```python
from build123d import *

# Parameters (mm, degrees)
CROQUIS1_R              = 2
CROQUIS1_R_2            = 3.5
CROQUIS1_R_3            = 4
CROQUIS1_W              = 30
CROQUIS1_H              = 3
CROQUIS1_R_4            = 1.5
CROQUIS1_W_2            = 15
CROQUIS1_H_2            = 55
SALIENTE_EXTRUIR4_DEPTH = 3


with BuildPart() as part:
    # Croquis1 → Saliente-Extruir4 (new body)
    with BuildSketch(Plane.XY):
        Polygon((-190, 67.5), (-190, -67.5), (-97.5, -67.5), (-97.5, -70.5), (-67.5, -70.5), (-67.5, -67.5), (-15, -67.5), (-15, -70.5), (15, -70.5), (15, -67.5), (67.5, -67.5), (67.5, -70.5), (97.5, -70.5), (97.5, -67.5), (190, -67.5), (190, 67.5), align=None)
        with Locations((-119.3, -56.25)):
            Circle(CROQUIS1_R, mode=Mode.SUBTRACT)
        with Locations((-170, -37.5)):
            Circle(CROQUIS1_R_2, mode=Mode.SUBTRACT)
        with Locations((-139.5, -47.5)):
            Circle(CROQUIS1_R_3, mode=Mode.SUBTRACT)
        with Locations((-119.3, -38.75)):
            Circle(CROQUIS1_R, mode=Mode.SUBTRACT)
        with Locations((-82.5, -29)):
            Rectangle(CROQUIS1_W, CROQUIS1_H, mode=Mode.SUBTRACT)
        with Locations((170, -37.5)):
            Circle(CROQUIS1_R_2, mode=Mode.SUBTRACT)
        with Locations((0, -29)):
            Rectangle(CROQUIS1_W, CROQUIS1_H, mode=Mode.SUBTRACT)
        with Locations((82.5, -29)):
            Rectangle(CROQUIS1_W, CROQUIS1_H, mode=Mode.SUBTRACT)
        with Locations((-22, 9.5)):
            Circle(CROQUIS1_R_4, mode=Mode.SUBTRACT)
        with Locations((0, 25)):
            Rectangle(CROQUIS1_W_2, CROQUIS1_H_2, mode=Mode.SUBTRACT)
        with Locations((-167.5, 39.5)):
            Circle(CROQUIS1_R_4, mode=Mode.SUBTRACT)
        Polygon((-180, 57.5), (-180, 64.5), (-155, 64.5), (-155, 57.5), (-163.4, 57.5), (-173.4, 57.5), align=None, mode=Mode.SUBTRACT)
        with Locations((-22, 45.5)):
            Circle(CROQUIS1_R_4, mode=Mode.SUBTRACT)
        Polygon((-19.6, 57.5), (-19.6, 64.5), (5.4, 64.5), (5.4, 57.5), (-3, 57.5), (-3, 54.5), (-13, 54.5), (-13, 57.5), align=None, mode=Mode.SUBTRACT)
        with Locations((167.5, 39.5)):
            Circle(CROQUIS1_R_4, mode=Mode.SUBTRACT)
        Polygon((155, 57.5), (155, 64.5), (180, 64.5), (180, 57.5), (171.6, 57.5), (161.6, 57.5), align=None, mode=Mode.SUBTRACT)
    extrude(amount=SALIENTE_EXTRUIR4_DEPTH)


solid = part.part
```
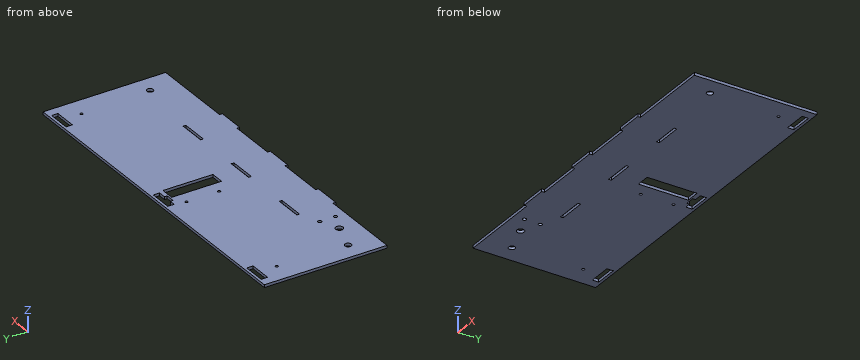
Could you check a few things on this model? Use its own coordinates, in mm. Coordinates: 2 decimals unless noted, no trailing zeros. Write each loop counter-clockwise with the first axis right and the second up, starting at its lowest first coordinate (ties: lowest second). Pieces come first, ordered by that corner, then holes. Notation, with made-up numbers: (6.5, 11.25) -> (49.5, 11.25) arc R13 cw to (49.5, 27.25) -> close; hole circle Ø2 at (-12.75, 3). An arc over 180 degrees is marked (long way). One line per question, with ' | ' between items. Start each with the question number.
1. If we section it at A-A (y = 24.5): Please give me the cut outline in (x, z).
2. If we section it at D-D (x = -106): Please give me the cut outline in (y, z).
3. Please list where these lines run through material, in increasing order: line 1 along Y through (x, z) = (-119.3, 0.75); line 2 along Y through (x, z) = (-170, 1.35); line 3 along Y through (x, z) = (-6, 1.2).
4. If we section it at C-C (y = -47.5): Please give me the cut outline in (x, z).
5. If we section it at B-B (z = 0.6): Count the separate pieces of the cut face and the enclosed holes in it, and give its area (3 significant figures).
6. Will these pins go through, and if not, where does the flat tip stop? P1, Ø1.5, axis at y = -68.5, z = 2, coming from the +X side; P2, Ø1, axis at x = -149.5, z = 1, coming from the -Y side.
Return value:
1) outline: (-190, 0) -> (-7.5, 0) -> (-7.5, 3) -> (-190, 3) -> close; (7.5, 0) -> (190, 0) -> (190, 3) -> (7.5, 3) -> close
2) outline: (-67.5, 0) -> (67.5, 0) -> (67.5, 3) -> (-67.5, 3) -> close
3) line 1: y = -67.5 to -58.25, -54.25 to -40.75, -36.75 to 67.5 | line 2: y = -67.5 to -41, -34 to 57.5, 64.5 to 67.5 | line 3: y = -70.5 to -30.5, -27.5 to -2.5, 52.5 to 54.5, 64.5 to 67.5
4) outline: (-190, 0) -> (-143.5, 0) -> (-143.5, 3) -> (-190, 3) -> close; (-135.5, 0) -> (190, 0) -> (190, 3) -> (-135.5, 3) -> close
5) separate pieces: 1 | enclosed holes: 16 | area: 49,700 mm²
6) P1: stops at x = 97.5 | P2: stops at y = -67.5
